For this review, take the finished solid that the model builds, in its own axes (mm). A direction names the side the tool comes from. Round coordinates to 2 decimals unless told otherwise and drop trailing zeros. Write each loop counter-clockwise with the first axis right and the second up, starting at its lowest first coordinate (ties: lowest second). Pieces come first, ordered by that corner, then holes. Notation, with made-up numbers: (41, 48.25) - (72, 48.25) arc R26 cw to (72, 63.25) - close; hole circle Ø10 at (5.5, 80.5). An arc over 180 degrees is marked (long way). Answer in a Markdown table with one row per item. Add a question column.
from build123d import *

# Parameters (mm, degrees)
SKETCH1_R           = 1
SKETCH1_R_2         = 3
SKETCH1_R_3         = 2.9
SKETCH1_R_4         = 1.575
BOSS_EXTRUDE3_DEPTH = 2.7


with BuildPart() as part:
    # Sketch1 → Boss-Extrude3 (new body)
    with BuildSketch(Plane.XY):
        Polygon((-45.972294428, -28.145904304), (-45.972294428, -25.445904304), (-15.292294428, -25.445904304), (-15.292294428, -28.145904304), (15.387705572, -28.145904304), (15.387705572, -25.445904304), (46.067705572, -25.445904304), (46.067705572, -28.145904304), (76.747705572, -28.145904304), (76.747705572, -25.445904304), (76.747705572, -23.145904304), (76.747705572, 12.854095696), (76.747705572, 110.140892261), (55.534502136, 131.354095696), (-55.439090993, 131.354095696), (-76.652294428, 110.140892261), (-76.652294428, 12.854095696), (-76.652294428, -23.145904304), (-76.652294428, -25.445904304), (-76.652294428, -28.145904304), align=None)
        with Locations((-21.25, -16.25)):
            Circle(SKETCH1_R, mode=Mode.SUBTRACT)
        with Locations((-27.5, -7.5)):
            Circle(SKETCH1_R_2, mode=Mode.SUBTRACT)
        with Locations((-21.25, 1.25)):
            Circle(SKETCH1_R, mode=Mode.SUBTRACT)
        with Locations((21.25, -16.25)):
            Circle(SKETCH1_R, mode=Mode.SUBTRACT)
        with Locations((27.5, -7.5)):
            Circle(SKETCH1_R_3, mode=Mode.SUBTRACT)
        with Locations((21.25, 1.25)):
            Circle(SKETCH1_R, mode=Mode.SUBTRACT)
        with Locations((0, 31.25)):
            Circle(SKETCH1_R_4, mode=Mode.SUBTRACT)
        with Locations((0, 12.75)):
            Circle(SKETCH1_R_4, mode=Mode.SUBTRACT)
        with Locations((-8.443747687, 17.125)):
            Circle(SKETCH1_R_4, mode=Mode.SUBTRACT)
        with Locations((-8.443747687, 26.875)):
            Circle(SKETCH1_R_4, mode=Mode.SUBTRACT)
        with Locations((8.443747687, 26.875)):
            Circle(SKETCH1_R_4, mode=Mode.SUBTRACT)
        with Locations((8.443747687, 17.125)):
            Circle(SKETCH1_R_4, mode=Mode.SUBTRACT)
        Polygon((-22.5, -3.5), (-14.5, 2.5), (14.5, 2.5), (22.5, -3.5), (22.5, -11.5), (14.5, -17.5), (0, -17.5), (-14.5, -17.5), (-22.5, -11.5), align=None, mode=Mode.SUBTRACT)
        Polygon((35.5, 57.5), (22.92, 57.5), (22.92, 54.8), (7.64, 54.8), (7.64, 57.5), (-7.64, 57.5), (-7.64, 54.8), (-22.92, 54.8), (-22.92, 57.5), (-35.5, 57.5), (-35.5, 65.68), (-38.2, 65.68), (-38.2, 76.56), (-35.5, 76.56), (-35.5, 87.44), (-38.2, 87.44), (-38.2, 98.32), (-35.5, 98.32), (-35.5, 106.5), (-22.92, 106.5), (-22.92, 109.2), (-7.64, 109.2), (-7.64, 106.5), (7.64, 106.5), (7.64, 109.2), (22.92, 109.2), (22.92, 106.5), (35.5, 106.5), (35.5, 98.32), (38.2, 98.32), (38.2, 87.44), (35.5, 87.44), (35.5, 76.56), (38.2, 76.56), (38.2, 65.68), (35.5, 65.68), align=None, mode=Mode.SUBTRACT)
    extrude(amount=BOSS_EXTRUDE3_DEPTH)


solid = part.part
Q1. Insertion check: pin 1 Ø1.2 at (x, y) = (-21.25, -16.25) entering from +Z; pin 2 Ø0.8 at (x, z) = (27.5, 1) entering from -Y. Each pin has a flat end and moves straight along its axis. Give the tip position at first contact, or say it passes through.
Q2. Add section B-B on x = 27.5. State the section outline as (y, z) points, then the cut area to 3 significant figures.
Q3. Draft analysis for pull direction X (two halves, no side actions). For faces 3 (the face through (30.266, -6.629, 1.331)), 4 (the face through (66.29, 120.6, 1.33)), 5 (the face through (-1, 53, 2.7)), 6 (the face through (-65.897, 120.896, 1.331)), state which applies: released by +X, released by -X, zero draft, split by the parting line, or undercut.
Q4. To check wall thickness, follow probe 1 along Y at (x, z) = (-27.5, 0.7); probe 2 along Y at (x, z) = (-38, 2.35); probe 3 along X at (y, z) = (95.5, 0.7). State the ranges of each line that lie inside material, in increasing order.
Q5. Add section D-D on x = -27.5. State the section outline as (y, z) points.
Q6. Add section C-C on y = -7.5. State the section outline as (x, z) points.
Q7. Tool access review of faces 1 (the face through (-1, 53, 0)), 2 (the face through (-18.556, -0.542, 1.331)): name each direction out of +Z, -Z, +X, -X, +Y, -Y from which nothing blocks a thin tool from reaching the whole face with its end or side.
Q8. Add section A-A on y = 73. State the section outline as (x, z) points, then the cut area to 3 significant figures.
Answer sheet:
| question | item | result |
|---|---|---|
| 1 | pin 1 | passes through |
| 1 | pin 2 | stops at y = -25.45 |
| 2 | outline | (-25.45, 0) - (-10.4, 0) - (-10.4, 2.7) - (-25.45, 2.7) - close; (-4.6, 0) - (57.5, 0) - (57.5, 2.7) - (-4.6, 2.7) - close; (106.5, 0) - (131.35, 0) - (131.35, 2.7) - (106.5, 2.7) - close |
| 2 | area | 275 mm² |
| 3 | face 3 | undercut |
| 3 | face 4 | released by +X |
| 3 | face 5 | zero draft |
| 3 | face 6 | released by -X |
| 4 | probe 1 | y = -25.45 to -10.5, -4.5 to 57.5, 106.5 to 131.35 |
| 4 | probe 2 | y = -25.45 to 65.68, 76.56 to 87.44, 98.32 to 131.35 |
| 4 | probe 3 | x = -76.65 to -38.2, 38.2 to 76.75 |
| 5 | outline | (-25.45, 0) - (-10.5, 0) - (-10.5, 2.7) - (-25.45, 2.7) - close; (-4.5, 0) - (57.5, 0) - (57.5, 2.7) - (-4.5, 2.7) - close; (106.5, 0) - (131.35, 0) - (131.35, 2.7) - (106.5, 2.7) - close |
| 6 | outline | (-76.65, 0) - (-30.5, 0) - (-30.5, 2.7) - (-76.65, 2.7) - close; (-24.5, 0) - (-22.5, 0) - (-22.5, 2.7) - (-24.5, 2.7) - close; (22.5, 0) - (24.6, 0) - (24.6, 2.7) - (22.5, 2.7) - close; (30.4, 0) - (76.75, 0) - (76.75, 2.7) - (30.4, 2.7) - close |
| 7 | face 1 | -Z, +X, -X, +Y, -Y |
| 7 | face 2 | +Z, -Z |
| 8 | outline | (-76.65, 0) - (-38.2, 0) - (-38.2, 2.7) - (-76.65, 2.7) - close; (38.2, 0) - (76.75, 0) - (76.75, 2.7) - (38.2, 2.7) - close |
| 8 | area | 208 mm² |
